Geometry check sheet. Reference: the model listing, model coordinates, mm. A direction names the side the tool comes from. Give positions to 0.01 mm unless a question says otherwise; leave off trailing zeros. Loops run counter-clockwise (first coordinate to the right, second up) from the corner with the lowest first, then second, coordinate; pieces in that order, holes last.
```python
from build123d import *

# Parameters (mm, degrees)
F1_DEPTH = 27
F3_DEPTH = 33
F4_W     = 1.5
F4_H     = 13
F5_DEPTH = 22.75
F6_W     = 16
F6_H     = 3
F7_DEPTH = 5


with BuildPart() as f1:
    # F0 (on Top) → F1 (new body)
    with BuildSketch(Plane.XY):
        Polygon((28.95, 33), (-29.5, 33), (-29.5, 0), (-6.5, 0), (-6.5, 13), (6.5, 13), (6.5, 0), (28.95, 0), align=None)
    extrude(amount=F1_DEPTH)

    # F2 (on face) → F3 (cut, through all)
    with BuildSketch(Plane.XZ):
        Polygon((28.95, 0), (28.95, 27), (9.974082, 27), align=None)
        Polygon((-29.5, 0), (-10.524082, 27), (-29.454212, 27), (-29.5, 27), align=None)
    extrude(amount=-F3_DEPTH, mode=Mode.SUBTRACT)

    # F4 (on face) → F5 (cut)
    with BuildSketch(Plane.XY.offset(27)):
        with Locations((-7.25, 6.5)):
            Rectangle(F4_W, F4_H)
        with Locations((7.25, 6.5)):
            Rectangle(F4_W, F4_H)
    extrude(amount=-F5_DEPTH, mode=Mode.SUBTRACT)

    # F6 (on face) → F7 (cut)
    with BuildSketch(Plane.XZ.offset(-13)):
        with Locations((0, 23.5)):
            Rectangle(F6_W, F6_H)
    extrude(amount=-F7_DEPTH, mode=Mode.SUBTRACT)


solid = f1.part
```
1) Sectioned sample at A-A on y = 8. Enter the section's corners in (x, z).
2) Sectioned sample at C-C on x = -4.5. Enter the section's corners in (y, z), plus the area to 3 significant figures.
3) Tool access check on faces 1 (the flat face through (0, 15, 22)), 2 (the flat face through (15, 0, 10)), 3 (the flat face through (7, 7, 4.25)), 4 (the flat face through (-6.5, 6, 2)). Record the directions out of +Z, -Z, +X, -X, +Y, -Y that give a thin tool (end or side, any length) a straight path to the whole face; none if there is none.
4) Depth check by flat-ended pin: P1, Ø1.5, axis at x = -3, z = 23, coming from the -Y side; P2, Ø5, axis at x = 14, y = 14, coming from the +Z side; P3, Ø6, axis at y = 19.5, z = 18.5, coming from the -X side. Enter the tip coordinate at first touch or a pass-through.
5) Mould release check, pull along X, two halves, no side actions. Record for faces 5 (the flat face through (0, 18, 24)), 6 (the flat face through (-20.145, 16.269, 13.311)), 7 (the flat face through (-7, 7, 4.25)), 8 (the flat face through (19.33, 16.27, 13.69)): +X half, -X half, draft (parallel to the pull), parting line (faces both ways), or undercut.
6) Scan lines: line 1 along Z through (x, y) = (-0.5, 15.5); line 2 along Y through (x, z) = (3.5, 9.75); line 3 along Z through (x, y) = (7.5, 11). Record each from-to range of solid material in increasing order.
7) Sectioned sample at D-D on z = 12.5. Enter the section's corners in (x, y), plus the area to 3 significant figures.
8) Sectioned sample at B-B on y = 17. Enter the section's corners in (x, z), plus the area to 3 significant figures.
Determined:
1. outline: (-29.5, 0) - (-6.5, 0) - (-6.5, 4.25) - (-8, 4.25) - (-8, 27) - (-10.52, 27) - close; (6.5, 0) - (28.95, 0) - (9.97, 27) - (8, 27) - (8, 4.25) - (6.5, 4.25) - close
2. outline: (13, 0) - (33, 0) - (33, 27) - (13, 27) - (13, 25) - (18, 25) - (18, 22) - (13, 22) - close
2. area: 525 mm2
3. face 1: -Y
3. face 2: +Z, -Z, +X, -X, -Y
3. face 3: +Z, -Y
3. face 4: +Z, -Z, -Y
4. P1: stops at y = 18
4. P2: stops at z = 24.83
4. P3: stops at x = -18.61
5. face 5: undercut
5. face 6: -X half
5. face 7: undercut
5. face 8: +X half
6. line 1: z = 0 to 22, 25 to 27
6. line 2: y = 13 to 33
6. line 3: z = 0 to 4.25
7. outline: (-20.71, 0) - (-8, 0) - (-8, 13) - (8, 13) - (8, 0) - (20.16, 0) - (20.16, 33) - (-20.71, 33) - close
7. area: 1,140 mm2
8. outline: (-29.5, 0) - (28.95, 0) - (9.97, 27) - (-10.52, 27) - close; hole (-8, 22) - (8, 22) - (8, 25) - (-8, 25) - close
8. area: 1,020 mm2
